Here's how the part is built. I have some questions about the finished solid (model axes, mm). A direction names the side the tool comes from. Coordinates: 2 decimals unless noted, no trailing zeros. Order: outer loops, then holes, each group sorted by start corner. A loop starts at its lowest first (then second) coordinate and runs counter-clockwise, first axis right, second up. Notation, with made-up numbers: (-11, 26) - (16, 26) arc R23 cw to (16, 59) - close; hole circle Ø10 at (69.25, 63.5). An arc over 180 degrees is marked (long way). Answer as CSV lines item,"result". Start each with the question number.
Q1. Suppose I cut it at A-A (z = 80). Please give me the cut outline in (x, y).
Q2. Suppose I cut it at B-B (x = -11.5). Please give me the cut outline in (y, z), then the cut area to 3 significant figures.
Q3. For faces 1 (the face through (-24, -23, 3)), 2 (the face through (-24, -3, 2)), 3 (the face through (-6.23, -22.04, 18.78)), 4 (the face through (-58.59, -9.35, 26.17)), 5 (the face through (-25.896, -2.465, 8.283)), which set-ups out of +Z, -Z, +X, -X, +Y, -Y let a thin tool reach every point of the face, with its end or its side?
Q4. Thinking about a two-plate mould opening in X: for faces 6 (the face through (-43.273, -12, 46)), 7 (the face through (-45.738, -2.535, -11.583)), 8 (the face through (-48.5, 0, 31.3)), which applies, released by +X, released by -X, zero draft, split by the parting line, or undercut?
Q5. Suppose I cut it at D-D (z = 29). Please give me the cut outline in (x, y), then the cut area to 3 significant figures.
Q6. I need wall thicknesses on line 1 (X direction, y = -19.25, z = 62); line 2 (Z direction, x = -41.5, y = -5.25); line 3 (X direction, y = -7, z = 26). Which ranges of each line are inside material? Lowest first, please.
Q7. For pin 1 Ø4.5 at (y, z) = (-13.5, 47.5) entering from +X; pin 2 Ø7.5 at (x, y) = (-15, -12) entering from -Z; pin 3 Ø4.5 at (y, z) = (-12.12, 85.41) entering from +X, each with a flat end and sliding along its axis, tell me the tip position at first contact or that it passes through.
from build123d import *

# Parameters (mm, degrees)
F1_DEPTH   = 25
F2_SIZE    = 5
F3_SIZE    = 5
F4_C1_SIZE = 5
F4_C2_SIZE = 5
F4_C3_SIZE = 5
F4_C4_SIZE = 5
F5_SIZE    = 5
F6_R       = 3.8134977221
F6_R_2     = 4.2636207358
F6_R_3     = 3.889016134
F6_R_4     = 3.7558552916
F6_R_5     = 4.5761931688
F6_R_6     = 1.7054444875
F7_DEPTH   = 2.5


with BuildPart() as f1:
    # F0 (on Front) → F1 (new body)
    with BuildSketch(Plane.XZ):
        Polygon((0, 0), (0, 21.6363706006), (-8.27272566, 30.5454584579), (-8.27272566, 10.8181868544), (-43.27272566, 10.8181868544), (-43.27272566, 0), align=None)
        Polygon((-43.27272566, -28.6363649917), (-43.27272566, 0), (-43.27272566, 10.8181868544), (-43.27272566, 82.0909227153), (-59.8181864452, 99.2727460619), (-59.8181864452, -10.8181790838), align=None)
    extrude(amount=F1_DEPTH)

    # F2
    f2_edges = [f1.edges().sort_by_distance(p)[0] for p in [
        (-25.772726, -25, 10.818187),
        (-21.636363, -25, 0),
    ]]
    chamfer(f2_edges, length=F2_SIZE)

    # F3
    f3_edges = [f1.edges().sort_by_distance(p)[0] for p in [
        (-25.772726, 0, 10.818187),
        (-21.636363, 0, 0),
    ]]
    chamfer(f3_edges, length=F3_SIZE)

    # F4: chamfer of 5 on 4 edges, made by hand

    # F4_c1
    f4_c1_edges = [f1.edges().sort_by_distance(p)[0] for p in [
        (-8.27272566, 0, 20.6818226561),
        (-8.27272566, 0, 8.3181868544),
    ]]
    chamfer(f4_c1_edges, length=F4_C1_SIZE)

    # F4_c2
    f4_c2_edges = [f1.edges().sort_by_distance(p)[0] for p in [
        (-8.27272566, -25, 20.6818226561),
        (-8.27272566, -25, 8.3181868544),
    ]]
    chamfer(f4_c2_edges, length=F4_C2_SIZE)

    # F4_c3
    f4_c3_edges = [f1.edges().sort_by_distance(p)[0] for p in [
        (0, 0, 13.3181853003),
    ]]
    chamfer(f4_c3_edges, length=F4_C3_SIZE)

    # F4_c4
    f4_c4_edges = [f1.edges().sort_by_distance(p)[0] for p in [
        (0, -25, 13.3181853003),
    ]]
    chamfer(f4_c4_edges, length=F4_C4_SIZE)

    # F5
    f5_edges = [f1.edges().sort_by_distance(p)[0] for p in [
        (-43.272726, 0, 46.454555),
        (-43.272726, 0, -14.318182),
        (-59.818186, 0, 44.227283),
        (-43.272726, -25, 46.454555),
        (-43.272726, -25, -14.318182),
        (-59.818186, -25, 44.227283),
    ]]
    chamfer(f5_edges, length=F5_SIZE)

    # F6 (on face) → F7 (cut)
    with BuildSketch(Plane(origin=(-59.8181864452, 0, 0), x_dir=(0, -1, 0), z_dir=(-1, 0, 0))):
        with Locations((12.1186533943, 85.4130089283)):
            Circle(F6_R)
        with Locations((12.1186533943, 65.2014911175)):
            Circle(F6_R_2)
        with Locations((12.1186533943, 45.3713275492)):
            Circle(F6_R_3)
        with Locations((12.1186533943, 23.6344132572)):
            Circle(F6_R_4)
        with Locations((12.1186533943, 6.4736939967)):
            Circle(F6_R_5)
        with Locations((12.1186533943, -4.9667861313)):
            Circle(F6_R_6)
    extrude(amount=-F7_DEPTH, mode=Mode.SUBTRACT)


solid = f1.part
Here are the results:
1,outline,"(-59.82, -20) - (-54.82, -25) - (-48.27, -25) - (-43.27, -20) - (-43.27, -5) - (-48.27, 0) - (-54.82, 0) - (-59.82, -5) - close"
2,outline,"(-25, 5) - (-20, 0) - (-5, 0) - (0, 5) - (0, 5.82) - (-5, 10.82) - (-20, 10.82) - (-25, 5.82) - close"
2,area,"220 mm²"
3,face 1,"-Z, +X, -Y"
3,face 2,"-Z, +X, +Y"
3,face 3,"+Z, -Y"
3,face 4,"-X"
3,face 5,"+Z, +Y"
4,face 6,"undercut"
4,face 7,"released by +X"
4,face 8,"zero draft"
5,outline,"(-59.82, -20) - (-54.82, -25) - (-48.27, -25) - (-43.27, -20) - (-43.27, -5) - (-48.27, 0) - (-54.82, 0) - (-59.82, -5) - close; (-8.27, -20) - (-6.84, -21.44) - (-6.84, -3.56) - (-8.27, -5) - close"
5,area,"387 mm²"
6,line 1,"x = -59.82 to -43.27"
6,line 2,"z = 0 to 10.82"
6,line 3,"x = -59.82 to -43.27, -8.27 to -4.05"
7,pin 1,"stops at x = -43.27"
7,pin 2,"stops at z = 0"
7,pin 3,"stops at x = -44.3"
